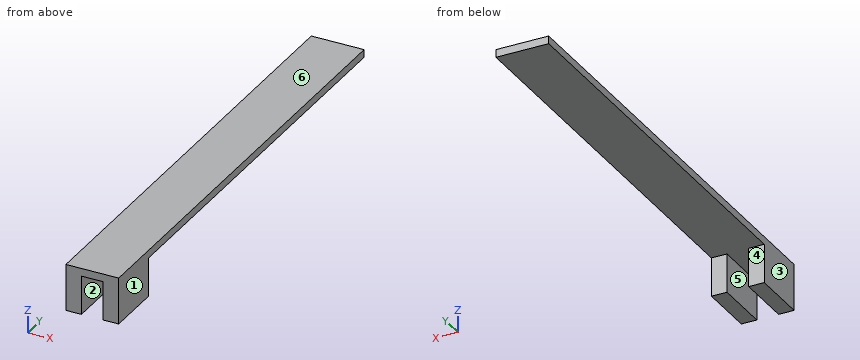
```python
from build123d import *

# Parameters (mm, degrees)
F0_W     = 2
F0_H     = 7.3
F1_DEPTH = 5
F2_W     = 6.8
F2_H     = 60
F3_DEPTH = 1


with BuildPart() as f1:
    # F0 (on Top) → F1 (new body)
    with BuildSketch(Plane.XY):
        with Locations((-2.4, 3.65)):
            Rectangle(F0_W, F0_H)
    extrude(amount=F1_DEPTH)



with BuildPart() as f1b:
    # F0 (on Top) → F1, piece 2 (new body)
    with BuildSketch(Plane.XY):
        with Locations((2.4, 3.65)):
            Rectangle(F0_W, F0_H)
    extrude(amount=F1_DEPTH)


with BuildPart() as f1_1:
    add(f1.part)

    add(f1b.part)  # F3 merges F1b
    # F2 (on face) → F3 (join)
    with BuildSketch(Plane.XY.offset(5)):
        with Locations((0, 30)):
            Rectangle(F2_W, F2_H)
    extrude(amount=F3_DEPTH)


solid = f1_1.part
```
The listing builds one solid part. Answer for the finished solid, in the listing's coordinates (mm). Face numbers are marked on the shaded views. A direction names the side the tool comes from. Give positions to 0.01 mm unless a question says otherwise; leave off trailing zeros. Order: outer loops, then holes, each group sorted by start corner. A loop starts at its lowest first (then second) coordinate and runs counter-clockwise, first axis right, second up. Notation, with made-up numbers: (69.5, -18.5) - (85.5, -18.5) arc R23 cw to (85.5, -5.5) - close; hole circle Ø8 at (78.5, 57). An arc over 180 degrees is marked (long way). Use one line per item in the form item = value. Start each with the question number.
(1) A cutting plane is placed at B-B, the plane x = 2.5. Write down the section's boundary in (y, z).
(2) A cutting plane is placed at D-D, the plane x = -0.5. Write down the section's boundary in (y, z).
(3) The mould has two halves that part along X. Classify the marked faces 1, 2 and 3: released by +X, released by -X, zero draft, split by the parting line, or undercut.
(4) For the marked faces 4, 5 and 6, determine the directions among +Z, -Z, +X, -X, +Y, -Y from which every point of the face is accessible in a straight line to the end or side of a thin tool.
(5) Consider line 1 (X direction, y = 7, z = 3.2); line 2 (Z direction, x = -1, y = 32.5); line 3 (Y direction, x = -1.75, z = 3.3). Determine where each line is inside the solid, lowest interval first. Write a range as from..to.
(6) A cutting plane is placed at A-A, the plane z = 2.05. Write down the section's boundary in (x, y).
(7) A cutting plane is placed at C-C, the plane y = 55. Write down the section's boundary in (x, z), then the cut area to 3 significant figures.
(8) Flat-ended cylindrical pins translate along their axes: pin 1 Ø1 at (x, z) = (-2, 2.5) entering from +Y; pin 2 Ø1 at (x, y) = (-0.5, 53.5) entering from -Z. Find the tip coordinate at first contact, or state that the pin passes through.
Ans:
q1.outline = (0, 0) - (7.3, 0) - (7.3, 5) - (60, 5) - (60, 6) - (0, 6) - close
q2.outline = (0, 5) - (60, 5) - (60, 6) - (0, 6) - close
q3.face_1 = released by +X
q3.face_2 = undercut
q3.face_3 = released by -X
q4.face_4 = -Z, +X, -X, +Y
q4.face_5 = -Z, +Y, -Y
q4.face_6 = +Z, +X, -X, +Y, -Y
q5.line_1 = -3.4..-1.4, 1.4..3.4
q5.line_2 = 5..6
q5.line_3 = 0..7.3
q6.outline = (-3.4, 0) - (-1.4, 0) - (-1.4, 7.3) - (-3.4, 7.3) - close; (1.4, 0) - (3.4, 0) - (3.4, 7.3) - (1.4, 7.3) - close
q7.outline = (-3.4, 5) - (3.4, 5) - (3.4, 6) - (-3.4, 6) - close
q7.area = 6.80 mm^2
q8.pin_1 = 7.3
q8.pin_2 = 5
